```python
from build123d import *

# Parameters (mm, degrees)
F0_W           = 60
F0_H           = 35
F1_DEPTH       = 20.5
F2_W           = 60
F2_H           = 8
F3_DEPTH       = 24
F5_D           = 5.5
F5_CBORE_D     = 9
F5_CBORE_DEPTH = 2
F7_D           = 4.5
F7_DEPTH       = 3
F7_TIP         = 1.3519363928


with BuildPart() as f1:
    # F0 (on Top) → F1 (new body)
    with BuildSketch(Plane.XY):
        Rectangle(F0_W, F0_H)
    extrude(amount=F1_DEPTH)

    # F2 (on face) → F3 (join)
    with BuildSketch(Plane.XY.offset(20.5)):
        with Locations((0, 13.5)):
            Rectangle(F2_W, F2_H)
    extrude(amount=F3_DEPTH)

    # F5 (through all)
    with Locations(Plane.XZ.offset(-9.5)):
        with Locations((0, 25.5)):
            CounterBoreHole(F5_D / 2, F5_CBORE_D / 2, F5_CBORE_DEPTH)

    # F7
    with Locations(Plane(origin=(0, 17.5, 0), x_dir=(-1, 0, 0), z_dir=(0, 1, 0))):
        with Locations((0, 15.5)):
            Hole(F7_D / 2, depth=F7_DEPTH)
            with Locations((0, 0, -(F7_DEPTH + F7_TIP / 2))):  # 118° drill point
                Cone(0, F7_D / 2, F7_TIP, mode=Mode.SUBTRACT)


solid = f1.part
```
The model under review builds one solid part; all positions refer to its coordinate system, in mm. A direction names the side the tool comes from. Give positions to 0.01 mm unless a question says otherwise; leave off trailing zeros. Order: outer loops, then holes, each group sorted by start corner. A loop starts at its lowest first (then second) coordinate and runs counter-clockwise, first axis right, second up. Notation, with made-up numbers: (-22, -12.5) - (5, -12.5) arc R7 ccw to (5, -6.5) - close; hole circle Ø11 at (-33.5, -31). An arc over 180 degrees is marked (long way). Use CSV: the item, a comma, the result in double quotes. Start each with the question number.
Q1. Clearance check with flat-ended pins moving along their axes: pin 1 Ø5 at (x, y) = (18.5, -9) entering from +Z; pin 2 Ø4.5 at (x, z) = (0, 25.5) entering from -Y; pin 3 Ø3.5 at (x, z) = (0, 15.5) entering from +Y; pin 4 Ø1.5 at (x, z) = (23.5, 38.5) entering from -Y. State where each tip first meets the part, or that it passes through.
Q2. The part is to be moulded in two halves that separate along X. For faces 1 (the flat face through (0, 14, 44.5)), 2 (the flat face through (30, 4, 12)), 3 (the conical face through (0.08, 13.38, 15.12)), say which applies: +X half, -X half, draft (parallel to the pull), parting line (faces both ways), or undercut.
Q3. We need section C-C, the plane y = -15. Write out the cut boundary in (x, z), and give its area (3 significant figures).
Q4. To check wall thickness, follow line 1 along Z through (x, y) = (0, 15); line 2 along Z through (x, y) = (0, 10); line 3 along Y through (x, z) = (-11, 23). State the ranges of each line that lie inside material, in increasing order. Write a range as [from, to].
Q5. We need section A-A, the plane z = 25.5. Write out the cut boundary in (x, y), and give its area (3 significant figures).
Q6. We need section B-B, the plane x = -7.5. Write out the cut boundary in (y, z).
Q7. Tool access review of faces 4 (the cylindrical face through (-0.59, 10.49, 29.96)), 5 (the cylindrical face through (-0.488, 15.979, 13.304)), 6 (the flat face through (0, -4, 20.5)): name each direction out of +Z, -Z, +X, -X, +Y, -Y from which nothing blocks a thin tool from reaching the whole face with its end or side.
Outcome:
1,pin 1,"stops at z = 20.5"
1,pin 2,"passes through"
1,pin 3,"stops at y = 14.2"
1,pin 4,"stops at y = 9.5"
2,face 1,"draft"
2,face 2,"+X half"
2,face 3,"undercut"
3,outline,"(-30, 0) - (30, 0) - (30, 20.5) - (-30, 20.5) - close"
3,area,"1,230 mm^2"
4,line 1,"z = [0, 13.25], [17.75, 22.75], [28.25, 44.5]"
4,line 2,"z = [0, 21], [30, 44.5]"
4,line 3,"y = [9.5, 17.5]"
5,outline,"(-30, 9.5) - (-4.5, 9.5) - (-4.5, 11.5) - (-2.75, 11.5) - (-2.75, 17.5) - (-30, 17.5) - close; (2.75, 11.5) - (4.5, 11.5) - (4.5, 9.5) - (30, 9.5) - (30, 17.5) - (2.75, 17.5) - close"
5,area,"429 mm^2"
6,outline,"(-17.5, 0) - (17.5, 0) - (17.5, 44.5) - (9.5, 44.5) - (9.5, 20.5) - (-17.5, 20.5) - close"
7,face 4,"-Y"
7,face 5,"+Y"
7,face 6,"+Z, +X, -X, -Y"
